```python
from build123d import *

# Parameters (mm, degrees)
F0_W      = 914.4
F0_H      = 25.4
F1_DEPTH  = 203.2
F2_T      = -3.175
F3_W      = 38.1
F3_H      = 38.1
F4_DEPTH  = 914.4
F5_W      = 406.4
F5_H      = 6.35
F6_DEPTH  = 914.4
F7_DEPTH  = 25.4
F8_DEPTH  = 25.4
F9_W      = 304.8
F9_H      = 400.05
F10_DEPTH = 0.254


with BuildPart() as f1:
    # F0 (on Front) → F1 (new body, symmetric)
    with BuildSketch(Plane.XZ):
        with Locations((5.9522092342, 25.7644668688)):
            Rectangle(F0_W, F0_H)
    extrude(amount=F1_DEPTH, both=True)

    # F2
    f2_openings = [f1.faces().sort_by_distance(p)[0] for p in [
        (5.952209, 0, 38.464467),
    ]]
    offset(amount=F2_T, openings=f2_openings)

    # F3 (on face) → F4 (join)
    with BuildSketch(Plane(origin=(0, 0, 13.0644668688), x_dir=(1, 0, 0), z_dir=(0, 0, -1))):
        with Locations((444.1022092342, 184.15)):
            Rectangle(F3_W, F3_H)
        with Locations((444.1022092342, -184.15)):
            Rectangle(F3_W, F3_H)
        with Locations((-432.1977907658, 184.15)):
            Rectangle(F3_W, F3_H)
        with Locations((-432.1977907658, -184.15)):
            Rectangle(F3_W, F3_H)
    extrude(amount=F4_DEPTH)

    # F5 (on face) → F6 (join, through all)
    with BuildSketch(Plane.YZ.offset(463.1522092342)):
        with Locations((0, -371.1105331312)):
            Rectangle(F5_W, F5_H)
    extrude(amount=-F6_DEPTH)

    # F7 (cut): a face of the model
    f7_faces = [f1.faces().sort_by_distance(p)[0] for p in [
        (-448.0727907658, 0, 27.3519668688),
    ]]
    extrude(f7_faces, amount=-F7_DEPTH, mode=Mode.SUBTRACT)

    # F8 (cut): a face of the model
    f8_faces = [f1.faces().sort_by_distance(p)[0] for p in [
        (459.9772092342, 0, 27.3519668688),
    ]]
    extrude(f8_faces, amount=-F8_DEPTH, mode=Mode.SUBTRACT)

    # F9 (on face) → F10 (join)
    with BuildSketch(Plane.XY.offset(16.2394668688)):
        with Locations((310.7522092342, 0)):
            Rectangle(F9_W, F9_H)
    extrude(amount=F10_DEPTH)


solid = f1.part
```
Geometry: final body of the model. Coordinates: model frame, mm. A direction names the side the tool comes from. Round coordinates to 2 decimals unless told otherwise and drop trailing zeros. Order: outer loops, then holes, each group sorted by start corner. A loop starts at its lowest first (then second) coordinate and runs counter-clockwise, first axis right, second up. Notation, with made-up numbers: M 58.25,68 L 65.25,68 A18 cw 65.25,80 Z; hole C 25,62 d10. An arc over 180 degrees is marked long. Use one line per item in the form item = value. Start each with the question number.
Q1. Mould query, pull axis Y, two halves, no side actions, for faces 6 (the face through (425.052, 184, -634)), 7 (the face through (-432, -165.1, -175)). Classes: +Y half, -Y half, draft (parallel to the pull), parting line (faces both ways), or undercut.
Q2. Cut plane D-D (x = 76). Return loops of the section in (y, z) (3 decimals).
Q3. Cut plane C-C (z = -129.5). Return loops of the section in (x, y).
Q4. Cut plane A-A (x = 202). Return loops of the section in (y, z) (3 decimals).
Q5. Material intervals for line 1 (Z direction, x = -177, y = 178); line 2 (Z direction, x = 257, y = -119.5); line 3 (X direction, y = 166.5, z = -858), sorted ascending. Write a range as [from, to].
Q6. Cut plane B-B (y = -90.5). Return loops of the section in (x, z), and give its area (3 significant figures).
Q7. Pin query (flat end, axial travel): pin 1 Ø5 at (x, y) = (-73.5, 150.5) entering from -Z; pin 2 Ø10 at (x, y) = (160.5, -66.5) entering from +Z; pin 3 Ø8 at (y, z) = (-63, -376.5) entering from -X. Return the tip coordinate at first contact, or that it passes through.
Q8. Access query for faces 1 (the face through (444, -165.1, -634)), 2 (the face through (463.152, 167, -429)), 3 (the face through (425.052, -184, -634)), 4 (the face through (444, 165.1, -175)), 5 (the face through (425.052, -184, -175)). Directions: +Z, -Z, +X, -X, +Y, -Y. A direction counts if a zero-diameter tool reaches every point of the face in a straight line with its end or side. Return the directions, or none.
Geometry results:
q1.face_6 = draft
q1.face_7 = undercut
q2.outline = M -203.2,-374.286 L 203.2,-374.286 L 203.2,-367.936 L -203.2,-367.936 Z; M -203.2,13.064 L 203.2,13.064 L 203.2,38.464 L 200.025,38.464 L 200.025,16.239 L -200.025,16.239 L -200.025,38.464 L -203.2,38.464 Z
q3.outline = M -451.25,-203.2 L -413.15,-203.2 L -413.15,-165.1 L -451.25,-165.1 Z; M -451.25,165.1 L -413.15,165.1 L -413.15,203.2 L -451.25,203.2 Z; M 425.05,-203.2 L 463.15,-203.2 L 463.15,-165.1 L 425.05,-165.1 Z; M 425.05,165.1 L 463.15,165.1 L 463.15,203.2 L 425.05,203.2 Z
q4.outline = M -203.2,-374.286 L 203.2,-374.286 L 203.2,-367.936 L -203.2,-367.936 Z; M -203.2,13.064 L 203.2,13.064 L 203.2,38.464 L 200.025,38.464 L 200.025,16.493 L -200.025,16.493 L -200.025,38.464 L -203.2,38.464 Z
q5.line_1 = [-374.29, -367.94], [13.06, 16.24]
q5.line_2 = [-374.29, -367.94], [13.06, 16.49]
q5.line_3 = [-451.25, -413.15], [425.05, 463.15]
q6.outline = M -451.25,-374.29 L 463.15,-374.29 L 463.15,-367.94 L -451.25,-367.94 Z; M -451.25,13.06 L 463.15,13.06 L 463.15,16.49 L 158.35,16.49 L 158.35,16.24 L -451.25,16.24 Z
q6.area = 8,790 mm^2
q7.pin_1 = -374.29
q7.pin_2 = 16.49
q7.pin_3 = -451.25
q8.face_1 = -Z, +X, -X
q8.face_2 = +Z, -Z, +X, +Y, -Y
q8.face_3 = -Z, +Y, -Y
q8.face_4 = +X, -X
q8.face_5 = +Y, -Y
